```python
from build123d import *

# Parameters (mm, degrees)
SKETCH_1_R      = 7.5
EXTRUDE_1_DEPTH = 20
SKETCH_2_W      = 200
SKETCH_2_H      = 8
EXTRUDE_2_DEPTH = 10
EXTRUDE_3_DEPTH = 7.5
FILLET_2_R      = 6
FILLET_3_R      = 2
FILLET_4_R      = 3


with BuildPart() as part:
    # 草图1 → 凸台-拉伸1 (new body)
    with BuildSketch(Plane.XY):
        Circle(SKETCH_1_R)
        Polygon((0, -4.618802154), (4, -2.309401077), (4, 2.309401077), (0, 4.618802154), (-4, 2.309401077), (-4, -2.309401077), align=None, mode=Mode.SUBTRACT)
    extrude(amount=EXTRUDE_1_DEPTH)

    # 草图2 → 凸台-拉伸2 (add)
    with BuildSketch(Plane(origin=(0, 0, 0), x_dir=(-1, 0, 0), z_dir=(0, 0, -1))):
        Rectangle(SKETCH_2_W, SKETCH_2_H)
    extrude(amount=EXTRUDE_2_DEPTH)

    # 草图3 → 凸台-拉伸3 (add, symmetric)
    with BuildSketch(Plane(origin=(0, 0, 0), x_dir=(1, 0, 0), z_dir=(0, 1, 0))):
        with BuildLine():
            Line((-100, 10), (-130, 18.038475773))
            ThreePointArc((-130, 18.038475773), (-132.710882753, 5), (-130, -8.038475773))
            Line((-130, -8.038475773), (-100, 0))
            Line((-100, 0), (-100, 10))
        make_face()
        with BuildLine():
            Line((100, 10), (100, 0))
            Line((100, 0), (130, -8.038475773))
            ThreePointArc((130, -8.038475773), (132.710882753, 5), (130, 18.038475773))
            Line((130, 18.038475773), (100, 10))
        make_face()
    extrude(amount=EXTRUDE_3_DEPTH, both=True)

    # 圆角2
    fillet_2_edges = [part.edges().sort_by_distance(p)[0] for p in [
        (-130, 0, -18.038475773),
        (-130, 0, 8.038475773),
        (130, 0, 8.038475773),
        (130, 0, -18.038475773),
    ]]
    fillet(fillet_2_edges, radius=FILLET_2_R)

    # 圆角3
    fillet_3_edges = [part.edges().sort_by_distance(p)[0] for p in [
        (-100, -7.5, -5),
        (-112.262976322, -7.5, -13.285854602),
        (-100, 7.5, -5),
        (-112.262976322, 7.5, -13.285854602),
        (100, -7.5, -5),
        (112.262976322, -7.5, 3.285854602),
        (100, 7.5, -5),
        (112.262976322, 7.5, 3.285854602),
        (-132.710882753, -7.5, -5),
        (-132.710882753, 7.5, -5),
        (-112.262976322, -7.5, 3.285854602),
        (-129.192011847, -7.5, 5.905318763),
        (-129.192011847, -7.5, -15.905318763),
        (-112.262976322, 7.5, 3.285854602),
        (-129.192011847, 7.5, 5.905318763),
        (-129.192011847, 7.5, -15.905318763),
        (112.262976322, -7.5, -13.285854602),
        (112.262976322, 7.5, -13.285854602),
        (132.710882753, -7.5, -5),
        (129.192011847, -7.5, 5.905318763),
        (129.192011847, -7.5, -15.905318763),
        (132.710882753, 7.5, -5),
        (129.192011847, 7.5, 5.905318763),
        (129.192011847, 7.5, -15.905318763),
    ]]
    fillet(fillet_3_edges, radius=FILLET_3_R)

    # 圆角4
    # the kernel refuses this fillet: 3 mm, written as the material it adds along each edge
    with BuildSketch(Plane(origin=(-6.42820323, -4, 0), x_dir=(0, 0, -1), z_dir=(1, 0, 0))) as fillet_4_piece_1_section:
        with BuildLine():
            CenterArc((FILLET_4_R, -FILLET_4_R), FILLET_4_R, 90, 90)
            Line((0, -FILLET_4_R), (0, 0))
            Line((0, 0), (FILLET_4_R, 0))
        make_face()
    fillet_4_piece_1 = extrude(amount=20.272492001, mode=Mode.PRIVATE)
    fillet_4_piece_1 = fillet_4_piece_1 & Plane(origin=(0, 0, -0.715829883), x_dir=(1, 0, 0), z_dir=(0, 0, -1)) * Cylinder(7.5, 53, mode=Mode.PRIVATE)
    fillet_4_piece_1 = split(fillet_4_piece_1, bisect_by=Plane(origin=(-2.485789841, -3.18363072, -0.715829883), z_dir=(-0.5000000000000003, -0.8660254037844387, 0)), keep=Keep.TOP, mode=Mode.PRIVATE)
    add(fillet_4_piece_1)
    with BuildSketch(Plane(origin=(-6.42820323, -4, 0), x_dir=(0, 0, -1), z_dir=(1, 0, 0))) as fillet_4_piece_2_section:
        with BuildLine():
            CenterArc((FILLET_4_R, -FILLET_4_R), FILLET_4_R, 90, 90)
            Line((0, -FILLET_4_R), (0, 0))
            Line((0, 0), (FILLET_4_R, 0))
        make_face()
    fillet_4_piece_2 = extrude(amount=20.272492001, mode=Mode.PRIVATE)
    fillet_4_piece_2 = fillet_4_piece_2 & Plane(origin=(0, 0, -0.715830721), x_dir=(1, 0, 0), z_dir=(0, 0, -1)) * Cylinder(7.5, 53, mode=Mode.PRIVATE)
    fillet_4_piece_2 = split(fillet_4_piece_2, bisect_by=Plane(origin=(2.485790597, -3.183630283, -0.715830721), z_dir=(0.4999999999999999, -0.8660254037844388, 0)), keep=Keep.TOP, mode=Mode.PRIVATE)
    add(fillet_4_piece_2)
    with BuildSketch(Plane(origin=(-13.84428877, -4, 0), x_dir=(0, 0, -1), z_dir=(1, 0, 0))) as fillet_4_piece_3_section:
        with BuildLine():
            CenterArc((FILLET_4_R, -FILLET_4_R), FILLET_4_R, 90, 90)
            Line((0, -FILLET_4_R), (0, 0))
            Line((0, 0), (FILLET_4_R, 0))
        make_face()
    fillet_4_piece_3 = extrude(amount=20.272492001, mode=Mode.PRIVATE)
    fillet_4_piece_3 = fillet_4_piece_3 & Plane(origin=(0, 0, -0.715829883), x_dir=(1, 0, 0), z_dir=(0, 0, -1)) * Cylinder(7.5, 53, mode=Mode.PRIVATE)
    fillet_4_piece_3 = split(fillet_4_piece_3, bisect_by=Plane(origin=(-2.485789841, -3.18363072, -0.715829883), z_dir=(-0.5000000000000003, -0.8660254037844387, 0)), keep=Keep.TOP, mode=Mode.PRIVATE)
    add(fillet_4_piece_3)
    with BuildSketch(Plane(origin=(-13.84428877, -4, 0), x_dir=(0, 0, -1), z_dir=(1, 0, 0))) as fillet_4_piece_4_section:
        with BuildLine():
            CenterArc((FILLET_4_R, -FILLET_4_R), FILLET_4_R, 90, 90)
            Line((0, -FILLET_4_R), (0, 0))
            Line((0, 0), (FILLET_4_R, 0))
        make_face()
    fillet_4_piece_4 = extrude(amount=20.272492001, mode=Mode.PRIVATE)
    fillet_4_piece_4 = fillet_4_piece_4 & Plane(origin=(0, 0, -0.715830721), x_dir=(1, 0, 0), z_dir=(0, 0, -1)) * Cylinder(7.5, 53, mode=Mode.PRIVATE)
    fillet_4_piece_4 = split(fillet_4_piece_4, bisect_by=Plane(origin=(2.485790597, -3.183630283, -0.715830721), z_dir=(0.4999999999999999, -0.8660254037844388, 0)), keep=Keep.TOP, mode=Mode.PRIVATE)
    add(fillet_4_piece_4)
    with BuildSketch(Plane(origin=(6.42820323, 4, 0), x_dir=(0, 0, -1), z_dir=(-1, 0, 0))) as fillet_4_piece_5_section:
        with BuildLine():
            CenterArc((FILLET_4_R, -FILLET_4_R), FILLET_4_R, 90, 90)
            Line((0, -FILLET_4_R), (0, 0))
            Line((0, 0), (FILLET_4_R, 0))
        make_face()
    fillet_4_piece_5 = extrude(amount=20.272492001, mode=Mode.PRIVATE)
    fillet_4_piece_5 = fillet_4_piece_5 & Plane(origin=(0, 0, -0.715829883), x_dir=(1, 0, 0), z_dir=(0, 0, -1)) * Cylinder(7.5, 53, mode=Mode.PRIVATE)
    fillet_4_piece_5 = split(fillet_4_piece_5, bisect_by=Plane(origin=(2.485789841, 3.18363072, -0.715829883), z_dir=(0.5, 0.8660254037844387, 0)), keep=Keep.TOP, mode=Mode.PRIVATE)
    add(fillet_4_piece_5)
    with BuildSketch(Plane(origin=(6.42820323, 4, 0), x_dir=(0, 0, -1), z_dir=(-1, 0, 0))) as fillet_4_piece_6_section:
        with BuildLine():
            CenterArc((FILLET_4_R, -FILLET_4_R), FILLET_4_R, 90, 90)
            Line((0, -FILLET_4_R), (0, 0))
            Line((0, 0), (FILLET_4_R, 0))
        make_face()
    fillet_4_piece_6 = extrude(amount=20.272492001, mode=Mode.PRIVATE)
    fillet_4_piece_6 = fillet_4_piece_6 & Plane(origin=(0, 0, -0.715830721), x_dir=(1, 0, 0), z_dir=(0, 0, -1)) * Cylinder(7.5, 53, mode=Mode.PRIVATE)
    fillet_4_piece_6 = split(fillet_4_piece_6, bisect_by=Plane(origin=(-2.485790597, 3.183630283, -0.715830721), z_dir=(-0.5000000000000001, 0.8660254037844387, 0)), keep=Keep.TOP, mode=Mode.PRIVATE)
    add(fillet_4_piece_6)
    with BuildSketch(Plane(origin=(13.84428877, 4, 0), x_dir=(0, 0, -1), z_dir=(-1, 0, 0))) as fillet_4_piece_7_section:
        with BuildLine():
            CenterArc((FILLET_4_R, -FILLET_4_R), FILLET_4_R, 90, 90)
            Line((0, -FILLET_4_R), (0, 0))
            Line((0, 0), (FILLET_4_R, 0))
        make_face()
    fillet_4_piece_7 = extrude(amount=20.272492001, mode=Mode.PRIVATE)
    fillet_4_piece_7 = fillet_4_piece_7 & Plane(origin=(0, 0, -0.715829883), x_dir=(1, 0, 0), z_dir=(0, 0, -1)) * Cylinder(7.5, 53, mode=Mode.PRIVATE)
    fillet_4_piece_7 = split(fillet_4_piece_7, bisect_by=Plane(origin=(2.485789841, 3.18363072, -0.715829883), z_dir=(0.5, 0.8660254037844387, 0)), keep=Keep.TOP, mode=Mode.PRIVATE)
    add(fillet_4_piece_7)
    with BuildSketch(Plane(origin=(13.84428877, 4, 0), x_dir=(0, 0, -1), z_dir=(-1, 0, 0))) as fillet_4_piece_8_section:
        with BuildLine():
            CenterArc((FILLET_4_R, -FILLET_4_R), FILLET_4_R, 90, 90)
            Line((0, -FILLET_4_R), (0, 0))
            Line((0, 0), (FILLET_4_R, 0))
        make_face()
    fillet_4_piece_8 = extrude(amount=20.272492001, mode=Mode.PRIVATE)
    fillet_4_piece_8 = fillet_4_piece_8 & Plane(origin=(0, 0, -0.715830721), x_dir=(1, 0, 0), z_dir=(0, 0, -1)) * Cylinder(7.5, 53, mode=Mode.PRIVATE)
    fillet_4_piece_8 = split(fillet_4_piece_8, bisect_by=Plane(origin=(-2.485790597, 3.183630283, -0.715830721), z_dir=(-0.5000000000000001, 0.8660254037844387, 0)), keep=Keep.TOP, mode=Mode.PRIVATE)
    add(fillet_4_piece_8)


solid = part.part
```
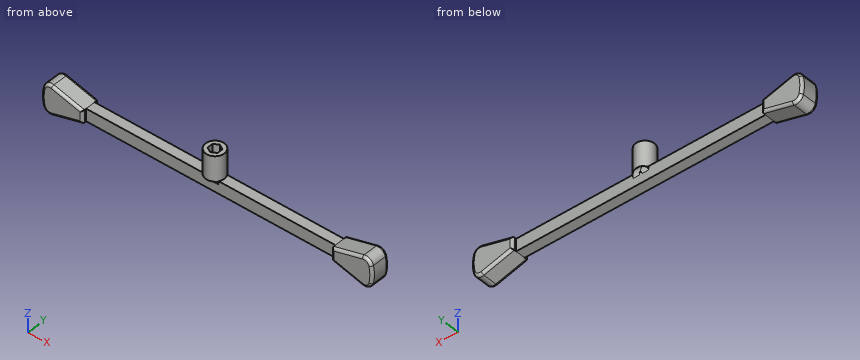
Verification items for the finished model (mm, model axes). Coordinates: 2 decimals unless noted, no trailing zeros. Loops run counter-clockwise (first coordinate to the right, second up) from the corner with the lowest first, then second, coordinate; pieces in that order, holes last. Notation, with made-up numbers: (-9.75, -9.75) - (20.25, -9.75) arc R9 cw to (20.25, -4.75) - close; hole circle Ø9 at (10, -3). An arc over 180 degrees is marked (long way). Put each result on its own line as item: value.
Item 1: Section check B-B (y = 0). Enter the section's corners in (x, z), then the cut area to 3 significant figures.
Conclusion:
outline: (-131.94, -12.07) arc R6 ccw to (-124.53, -16.57) - (-100, -10) - (100, -10) - (124.53, -16.57) arc R6 ccw to (131.94, -12.07) arc R32.71 ccw to (131.94, 2.07) arc R6 ccw to (124.53, 6.57) - (100, 0) - (7.5, 0) - (7.5, 20) - (4, 20) - (4, 0) - (-4, 0) - (-4, 20) - (-7.5, 20) - (-7.5, 0) - (-100, 0) - (-124.53, 6.57) arc R6 ccw to (-131.94, 2.07) arc R32.71 ccw to start
area: 3,290 mm2
Item 2: Section check C-C (x = 39.5). Enter the section's corners in (y, z), then the cut area to 3 significant figures.
Conclusion:
outline: (-4, -10) - (4, -10) - (4, 0) - (-4, 0) - close
area: 80.0 mm2
Item 3: Section check A-A (z = 16). Enter the section's corners in (x, y).
Conclusion:
outline: circle Ø15 at (0, 0); hole (-4, -2.31) - (0, -4.62) - (4, -2.31) - (4, 2.31) - (0, 4.62) - (-4, 2.31) - close
Item 4: Gauge pin test, flat ends, axial feed: pin 1 Ø0.8 at (y, z) = (5, -4.5) entering from -X; pin 2 Ø1.5 at (y, z) = (-0.5, -12.5) entering from -X; pin 3 Ø4 at (y, z) = (3.5, -9) entering from -X. Record the tip position at first contact, or that the pin passes through.
Conclusion:
pin 1: stops at x = -132.71
pin 2: stops at x = -132.01
pin 3: stops at x = -132.65
Item 5: Scan lines: line 1 along Z through (x, y) = (-74, -1.25); line 2 along X through (y, z) = (-0.25, 17); line 3 along X through (y, z) = (-2, 12). Record each from-to range of solid material in increasing order.
Conclusion:
line 1: z = -10 to 0
line 2: x = -7.5 to -4, 4 to 7.5
line 3: x = -7.23 to -4, 4 to 7.23
